from build123d import *

# Parameters (mm, degrees)
SKETCH1_R           = 4.85
SKETCH1_R_2         = 4
BOSS_EXTRUDE1_DEPTH = 52.5
SKETCH2_R           = 3.9
BOSS_EXTRUDE2_DEPTH = 8
SKETCH3_R           = 4.85
BOSS_EXTRUDE3_DEPTH = 2
CHAMFER1_SIZE       = 4
SKETCH4_R           = 4.85
BOSS_EXTRUDE4_DEPTH = 107
SKETCH5_R           = 4
CUT_EXTRUDE1_DEPTH  = 14
CHAMFER2_SIZE       = 3.9


with BuildPart() as part:
    # Sketch1 → Boss-Extrude1 (new body, symmetric)
    with BuildSketch(Plane(origin=(0, 0, 0), x_dir=(1, 0, 0), z_dir=(0, 1, 0))):
        Circle(SKETCH1_R)
        Circle(SKETCH1_R_2, mode=Mode.SUBTRACT)
    extrude(amount=BOSS_EXTRUDE1_DEPTH, both=True)



with BuildPart() as body_2:
    # Sketch2 → Boss-Extrude2 (new body)
    with BuildSketch(Plane(origin=(0, 52.5, 0), x_dir=(1, 0, 0), z_dir=(0, 1, 0))):
        Circle(SKETCH2_R)
    extrude(amount=BOSS_EXTRUDE2_DEPTH)


with BuildPart() as part_1:
    add(part.part)

    add(body_2.part)  # Boss-Extrude3 merges body 2
    # Sketch3 → Boss-Extrude3 (add)
    with BuildSketch(Plane(origin=(0, 52.5, 0), x_dir=(1, 0, 0), z_dir=(0, 1, 0))):
        Circle(SKETCH3_R)
    extrude(amount=BOSS_EXTRUDE3_DEPTH)

    # Chamfer1
    chamfer1_edges = [part_1.edges().sort_by_distance(p)[0] for p in [
        (-4, 52.5, 0),
    ]]
    chamfer(chamfer1_edges, length=CHAMFER1_SIZE)

    # Sketch4 → Boss-Extrude4 (add)
    with BuildSketch(Plane.XZ.offset(52.5)):
        Circle(SKETCH4_R)
    extrude(amount=-BOSS_EXTRUDE4_DEPTH)

    # Sketch5 → Cut-Extrude1 (cut)
    with BuildSketch(Plane.XZ.offset(52.5)):
        Circle(SKETCH5_R)
    extrude(amount=-CUT_EXTRUDE1_DEPTH, mode=Mode.SUBTRACT)

    # Chamfer2
    chamfer2_edges = [part_1.edges().sort_by_distance(p)[0] for p in [
        (-4, -38.5, 0),
    ]]
    chamfer(chamfer2_edges, length=CHAMFER2_SIZE)


solid = part_1.part
Here's how the part is built. I have some questions about the finished solid (model axes, mm). A direction names the side the tool comes from. Round coordinates to 2 decimals unless told otherwise and drop trailing zeros. Order: outer loops, then holes, each group sorted by start corner. A loop starts at its lowest first (then second) coordinate and runs counter-clockwise, first axis right, second up. Notation, with made-up numbers: M 11,62 L 35,62 A29 ccw 35,101 Z; hole C 20.25,-0.75 d3. An arc over 180 degrees is marked long. Return JSON: item names as keys, results as strings. Group by question number.
1. I'm going to push flat-ended pins straight in: pin 1 Ø1 at (x, y) = (1, -12) entering from -Z; pin 2 Ø5 at (y, z) = (-3.5, 4) entering from -X. Where does each tip first touch, or does it pass through?
2. If we mould it in two halves opening along X, with no side actions, what happens to faces 1 (the face through (4.626, 0.251, -1.457)), 2 (the face through (-2, -52.5, -4)), 3 (the face through (-0.917, -39.556, -0.703))? For each: pulls with the +X half, pulls with the -X half, needs draft (parallel to the pull), parting line crosses it, or undercut.
3. Please list where these lines run through material, in increasing order: probe 1 along Z at (x, y) = (0, -46); probe 2 along Z at (x, y) = (1, -44); probe 3 along Y at (x, z) = (4.25, 1.25).
4. On a 3-axis mill with a long thin cutter (end or side, diameter ignored), from which of +Z, -Z, +X, -X, +Y, -Y can I reach the whole of each face in a straight line? I mean faces 4 (the face through (-2.87, 57.46, -2.64)), 5 (the face through (0, 60.5, 0)), 6 (the face through (-0.867, -47.521, -3.905)). Say none if no direction works.
5. If we section it at A-A on y = 1: List the corners of the cut face in (x, z) for me, then the cut area to 3 significant figures.
Reply:
{
 "1": {"pin 1": "z = -4.82", "pin 2": "x = -4.61"},
 "2": {"face 1": "parting line crosses it", "face 2": "needs draft", "face 3": "undercut"},
 "3": {"probe 1": "-4.85 to -4, 4 to 4.85", "probe 2": "-4.75 to -3.87, 3.87 to 4.75", "probe 3": "-52.5 to 54.5"},
 "4": {"face 4": "+Y", "face 5": "+Z, -Z, +X, -X, +Y", "face 6": "-Y"},
 "5": {"outline": "C 0,0 d9.7", "area": "73.9 mm^2"}
}
